```python
from build123d import *

# Parameters (mm, degrees)
F0_W     = 290
F0_H     = 290
F1_DEPTH = 500
F3_DEPTH = 795
F5_DEPTH = 770


with BuildPart() as f1:
    # F0 (on Front) → F1 (new body)
    with BuildSketch(Plane.XZ):
        with Locations((145, 145)):
            Rectangle(F0_W, F0_H)
    extrude(amount=F1_DEPTH)

    # F2 (on face) → F3 (cut)
    with BuildSketch(Plane.XZ):
        with BuildLine():
            ThreePointArc((18.21568, 290), (211.733128, 199.092972), (289.675921, 0))
            Line((289.675921, 0), (290, 0))
            Line((290, 0), (290, 290))
            Line((290, 290), (18.21568, 290))
        make_face()
    extrude(amount=F3_DEPTH, mode=Mode.SUBTRACT)

    # F4 (on face) → F5 (cut)
    with BuildSketch(Plane.XZ.offset(500)):
        with BuildLine():
            Line((0, 0), (282.123595, 0))
            ThreePointArc((282.123595, 0), (199.483979, 199.530675), (0, 282.282948))
            Line((0, 282.282948), (0, 0))
        make_face()
    extrude(amount=-F5_DEPTH, mode=Mode.SUBTRACT)


solid = f1.part
```
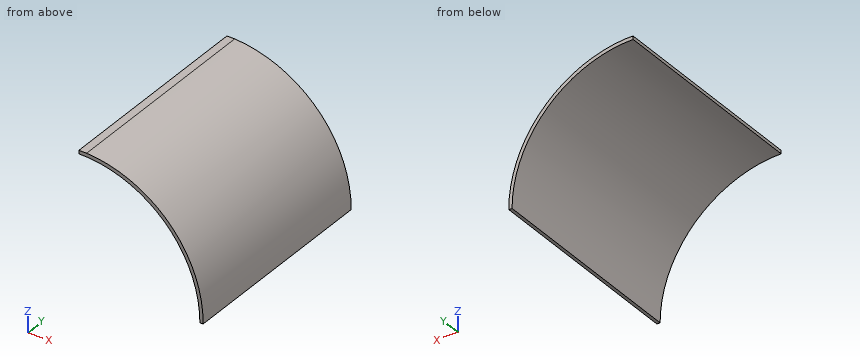
Source: CAD feature listing. Evaluate the final solid. Frame: model axes, mm. Round coordinates to 2 decimals unless told otherwise and drop trailing zeros. Loops run counter-clockwise (first coordinate to the right, second up) from the corner with the lowest first, then second, coordinate; pieces in that order, holes last.
1. Section query A-A on y = -186. Output: boundary loops of the cut face in (x, z), and give its area (3 significant figures).
2. Section query C-C on x = 233. Output: boundary loops of the cut face in (y, z).
3. Ray query, L1, parallel to X at y = -396, z = 13; L2, parallel to Z at x = 168.5, y = -418; L3, parallel to X at y = -70.5, z = 69. Return the intervals inside material, ascending.
4. Contact query for flat-ended pins moving along their axis: pin 1 (12 mm diameter, centred on y = -234.5, z = 102.5, fed in from -X); pin 2 (1.5 mm diameter, centred on x = 244.5, y = -217, fed in from +Z); pin 3 (1.5 mm diameter, centred on y = -329, z = 184.5, fed in from +X). Output: stop coordinate, or through.
Answers below:
1. outline: (0, 282.28) arc R282.34 cw to (282.12, 0) - (289.68, 0) arc R288.76 ccw to (18.22, 290) - (0, 290) - close
1. area: 3,730 mm2
2. outline: (-500, 159.08) - (0, 159.08) - (0, 173.58) - (-500, 173.58) - close
3. L1: x = 281.82 to 289.46
3. L2: z = 226.33 to 236.92
3. L3: x = 273.55 to 281.74
4. pin 1: stops at x = 260.42
4. pin 2: stops at z = 158.02
4. pin 3: stops at x = 225.11
